Check sheet for the modelled part. Datum: model origin and axes. Units: mm. Face numbers are marked on the shaded views. A direction names the side the tool comes from. Coordinates: 2 decimals unless noted, no trailing zeros. Loops run counter-clockwise (first coordinate to the right, second up) from the corner with the lowest first, then second, coordinate; pieces in that order, holes last. Notation, with made-up numbers: M 74,77.25 L 99,77.25 A14 ccw 99,102.25 Z; hole C 14.5,17 d1. An arc over 180 degrees is marked long. Use CSV: the item, a comma, the result in double quotes. Start each with the question number.
(1) Draft check along Y on the marked faces 3, 4, 5 and 6. Enter one of: pulls with the +Y half, pulls with the -Y half, needs draft (parallel to the pull), parting line crosses it, or undercut.
(2) Section check B-B on x = -197. Record the cut outline in (y, z), and give its area (3 significant figures).
(3) Section check A-A on z = -78.5. Record the cut outline in (x, y), and give its area (3 significant figures).
(4) Scan lines: line 1 (Y direction, x = -99, z = -47); line 2 (X direction, y = -93, z = -56.5); line 3 (Z direction, x = 262.5, y = 186). Record each from-to range of solid material in increasing order.
(5) Section check C-C on y = 415.5. Record the cut outline in (x, z).
(6) Go/stop test with a flat-tipped pin: pin 1 Ø1.5 at (x, y) = (232, 277) entering from +Z. Record where the tip stops, or that it passes through.
(7) Set-up check for the marked faces 1 and 2: record each of +Z, -Z, +X, -X, +Y, -Y from which the full face is reachable in a straight line by a thin tool's end or side.
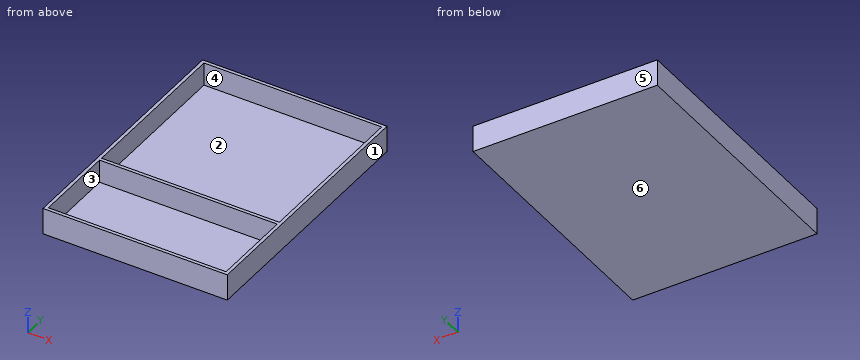
from build123d import *

# Parameters (mm, degrees)
F0_W     = 711.2
F0_H     = 990.6
F0_W_2   = 685.8
F0_H_2   = 317.5
F0_H_3   = 635
F0_H_4   = 12.7
F1_DEPTH = 101.6
F2_DEPTH = 88.9


with BuildPart() as f1:
    # F0 (on Top) → F1 (new body)
    with BuildSketch(Plane.XY):
        Rectangle(F0_W, F0_H)
        Polygon((342.9, -482.6), (-342.9, -482.6), (-342.9, -165.1), (-342.9, -152.4), (-342.9, 482.6), (342.9, 482.6), (342.9, -152.4), (342.9, -165.1), align=None, mode=Mode.SUBTRACT)
        with Locations((0, -323.85)):
            Rectangle(F0_W_2, F0_H_2)
        with Locations((0, 165.1)):
            Rectangle(F0_W_2, F0_H_3)
        with Locations((0, -158.75)):
            Rectangle(F0_W_2, F0_H_4)
    extrude(amount=-F1_DEPTH)

    # F0 (on Top) → F2 (cut, through all)
    with BuildSketch(Plane.XY):
        with Locations((0, 165.1)):
            Rectangle(F0_W_2, F0_H_3)
        with Locations((0, -323.85)):
            Rectangle(F0_W_2, F0_H_2)
    extrude(amount=-F2_DEPTH, mode=Mode.SUBTRACT)


solid = f1.part
Outcome:
1,face 3,"undercut"
1,face 4,"undercut"
1,face 5,"pulls with the +Y half"
1,face 6,"needs draft"
2,outline,"M -495.3,-101.6 L 495.3,-101.6 L 495.3,0 L 482.6,0 L 482.6,-88.9 L -152.4,-88.9 L -152.4,0 L -165.1,0 L -165.1,-88.9 L -482.6,-88.9 L -482.6,0 L -495.3,0 Z"
2,area,"16,000 mm²"
3,outline,"M -355.6,-495.3 L 355.6,-495.3 L 355.6,495.3 L -355.6,495.3 Z; hole M -342.9,-482.6 L 342.9,-482.6 L 342.9,-165.1 L -342.9,-165.1 Z; hole M -342.9,-152.4 L 342.9,-152.4 L 342.9,482.6 L -342.9,482.6 Z"
3,area,"51,300 mm²"
4,line 1,"y = -495.3 to -482.6, -165.1 to -152.4, 482.6 to 495.3"
4,line 2,"x = -355.6 to -342.9, 342.9 to 355.6"
4,line 3,"z = -101.6 to -88.9"
5,outline,"M -355.6,-101.6 L 355.6,-101.6 L 355.6,0 L 342.9,0 L 342.9,-88.9 L -342.9,-88.9 L -342.9,0 L -355.6,0 Z"
6,pin 1,"stops at z = -88.9"
7,face 1,"+Z, -Z, +X, +Y, -Y"
7,face 2,"+Z"
